Autodesk Fusion 360 part; units mm, degrees
sketch "Esquisse1" plane through (0, 0, 0) normal (0, 0, 1) x (1, 0, 0)
sketch "Esquisse2" plane through (0, 0, 0) normal (0, 0, 1) x (1, 0, 0)
  circle A0 centre (0, 0) radius 3.865
  line L0 (10, -10) -> (-10, -10)
  line L1 (-10, -10) -> (-10, 10)
  line L2 (-10, 10) -> (10, 10)
  line L3 (10, 10) -> (10, -10)
  dimension "d2" = 7.73
extrude "Extrusion1" add sketch "Esquisse2" along normal blind 20
sketch "Esquisse3" plane through (0, 10, 0) normal (0, 1, 0) x (-1, 0, 0)
  line L0 (-10, 0) -> (10, 0)
  line L1 (10, 0) -> (10, 20)
  line L2 (10, 20) -> (-10, 20)
  line L3 (-10, 20) -> (-10, 0)
sketch "Esquisse4" plane through (0, 0, 20) normal (0, 0, 1) x (-1, 0, 0)
  circle A0 centre (0, 0) radius 3.865
  line L0 (-10, -10) -> (10, -10)
  line L1 (10, -10) -> (10, 10)
  line L2 (10, 10) -> (-10, 10)
  line L3 (-10, 10) -> (-10, -10)
  line L4 (0, -7.4) -> (2.8, -7.4)
  line L5 (2.8, -7.4) -> (2.8, -5)
  line L6 (2.8, -5) -> (-2.8, -5)
  line L7 (-2.8, -5) -> (-2.8, -7.4)
  line L8 (-2.8, -7.4) -> (0, -7.4)
  dimension "d12" = 2.8
  dimension "d13" = 5.6
ref_plane "Plan de construction1" through (0, 0, 20) normal (0, 1, 0) x (-1, 0, 0)
sketch "Esquisse5" plane through (0, 0, 20) normal (0, 1, 0) x (-1, 0, 0)
  line L0 (0, 0) -> (0, -20)
  line L1 (-10, -10) -> (10, -10)
  line L2 (0, -6.8) -> (-2.7713, -8.4)
  line L3 (-2.7713, -8.4) -> (-2.7713, -11.6)
  line L4 (-2.7713, -11.6) -> (0, -13.2)
  line L5 (0, -13.2) -> (2.7713, -11.6)
  line L6 (2.7713, -11.6) -> (2.7713, -8.4)
  line L7 (2.7713, -8.4) -> (0, -6.8)
  point P0 (0, -10)
  dimension "d6" = 3.2
extrude "Extrusion2" cut sketch "Esquisse5" along normal blind 2.4 from surface at 5
extrude "Extrusion3" cut sketch "Esquisse4" against normal blind 9 contours L4 L5 L6 L7 L8
sketch "Esquisse6" plane through (0, 10, 0) normal (0, 1, 0) x (-1, 0, 0)
  circle A0 centre (0, 10) radius 1.625
  dimension "d16" = 3.25
extrude "Extrusion4" cut sketch "Esquisse6" against normal blind 10
sketch "Esquisse7" plane through (0, -10, 0) normal (0, -1, 0) x (1, 0, 0)
  line L0 (-10, 0) -> (10, 0)
  line L1 (10, 0) -> (10, 20)
  line L2 (10, 20) -> (-10, 20)
  line L3 (-10, 20) -> (-10, 0)
  line L4 (5, 15) -> (-5, 15)
  line L5 (-5, 15) -> (-5, 5)
  line L6 (-5, 5) -> (5, 5)
  line L7 (5, 5) -> (5, 15)
  line L8 (5, 15) -> (-5, 5) construction
  line L9 (-5, 15) -> (5, 5) construction
  point P0 (0, 10)
  dimension "d19" = 10
  dimension "d20" = 10
extrude "Extrusion5" add sketch "Esquisse7" along normal blind 70 contours L4 L5 L6 L7
sketch "Esquisse8" plane through (0, 0, 15) normal (0, 0, 1) x (-1, 0, 0)
  line L0 (-5, 10) -> (5, 10)
  line L1 (5, 10) -> (5, 80)
  line L2 (5, 80) -> (-5, 80)
  line L3 (-5, 80) -> (-5, 10)
  line L4 (5, 80) -> (-5, 80)
  line L5 (-5, 80) -> (-5, 75)
  line L6 (-5, 75) -> (5, 75)
  line L7 (5, 75) -> (5, 80)
  line L8 (-5, 75) -> (5, 75)
  line L9 (5, 75) -> (5, 70)
  line L10 (5, 70) -> (-5, 70)
  line L11 (-5, 70) -> (-5, 75)
extrude "Extrusion6" cut sketch "Esquisse8" against normal blind 3 contours L1 L3 L6 L8 L9 L10 L11
extrude "Extrusion7" add 1 faces at (-1.6667, -33.3333, 5) along direction (0, 0, -1) blind 5
extrude "Extrusion8" cut 2 faces at (1.6667, -50, 15) (1.6667, -76.6667, 15) along direction (0, 0, -1) blind 5
extrude "Extrusion9" cut 1 faces at (-1.6667, -71.6667, 12) along direction (0, 0, -1) blind 5
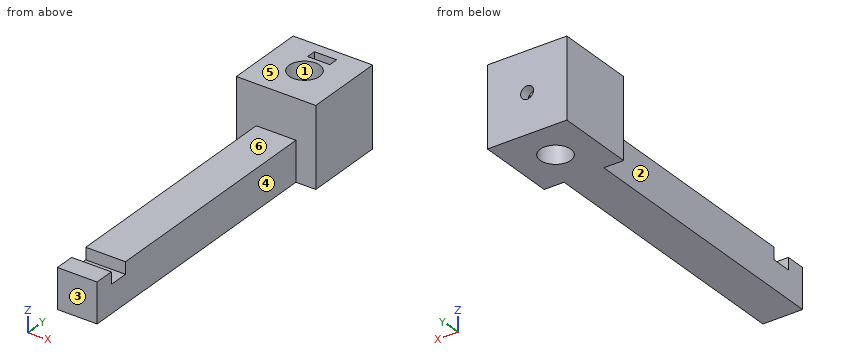
Here's how the part is built. I have some questions about the finished solid (model axes, mm). Face numbers are marked on the shaded views. A direction names the side the tool comes from. Coordinates: 2 decimals unless noted, no trailing zeros. Write each loop counter-clockwise with the first axis right and the second up, starting at its lowest first coordinate (ties: lowest second). Pieces come first, ordered by that corner, then holes.
1) Thinking about a two-plate mould opening in X: for the marked faces 1, 2 and 3, which applies, +X half, -X half, draft (parallel to the pull), parting line (faces both ways), or undercut?
Filled in:
face 1: undercut
face 2: -X half
face 3: draft
2) Which directions (+Z, -Z, +X, -X, +Y, -Y) give clear straight access to the entire face, cutting with the end or side of a thin tool? Please do the marked faces 4, 5 and 6.
Filled in:
face 4: +Z, -Z, +X, -Y
face 5: +Z, +X, -X, +Y, -Y
face 6: +Z, +X, -X, -Y
3) If we section it at C-C (z = 15): List the corners of the cut face in (x, y) for me (3 decimals).
Filled in:
outline: (-10, -10) - (10, -10) - (10, 10) - (-10, 10) - close; hole circle Ø7.73 at (0, 0); hole (-2.8, 5) - (2.8, 5) - (2.8, 7.4) - (-2.8, 7.4) - close
4) If we section it at A-A (z = 3.25): List the corners of the cut face in (x, y) for me (3 decimals), plus the area to 3 significant figures.
Filled in:
outline: (-10, -10) - (-5, -10) - (-5, -80) - (5, -80) - (5, -10) - (10, -10) - (10, 10) - (-10, 10) - close; hole circle Ø7.73 at (0, 0)
area: 1,050 mm2
5) I'm going to push flat-ended pins straight in: pin 1 (5.5 mm diameter, centred on x = 0, y = -78.5, fed in from +Z); pin 2 (6 mm diameter, centred on x = 1, z = 13.5, fed in from -Y); pin 3 (11 mm diameter, centred on y = -53.5, z = 5.5, fed in from -X); pin 4 (1 mm diameter, centred on x = 7, y = -50, fed in from -Z). Where does each tip first touch, or does it pass through?
Filled in:
pin 1: stops at z = 10
pin 2: stops at y = -10
pin 3: stops at x = -5
pin 4: passes through
6) If I drill on line 1 (Y direction, x = 0, z = 7.75) (3 decimals); line 2 (Y direction, x = -3.5, z = 9.25); line 3 (Z direction, x = 0, y = 8.2) (3 decimals), over which ranges is the centre line in solid material (lowest first)?
Filled in:
line 1: y = -80 to -75, -70 to -3.865, 3.865 to 5, 7.4 to 10
line 2: y = -80 to -75, -70 to -1.64, 1.64 to 10
line 3: z = 0 to 8.375, 11.625 to 20
7) If we section it at B-B (y = 0): List the corners of the cut face in (x, z) for me (3 decimals).
Filled in:
outline: (-10, 0) - (-3.865, 0) - (-3.865, 20) - (-10, 20) - close; (3.865, 0) - (10, 0) - (10, 20) - (3.865, 20) - close
8) If we section it at D-D (y = -66): List the corners of the cut face in (x, z) for me.
Filled in:
outline: (-5, 0) - (5, 0) - (5, 10) - (-5, 10) - close
